Source: CAD feature listing. Evaluate the final solid. Frame: model axes, mm. Face numbers are marked on the shaded views. Coordinates: 2 decimals unless noted, no trailing zeros. Loops run counter-clockwise (first coordinate to the right, second up) from the corner with the lowest first, then second, coordinate; pieces in that order, holes last.
Item 1: Line query: probe 1 along Y at (x, z) = (0, 14.75); probe 2 along Y at (x, z) = (0, 10.75); probe 3 along Y at (x, z) = (-3.5, 9.25). Output: solid intervals per line, ascending.
Item 2: Pull-direction query (Y, two-part tool) for the marked faces 1, 2, 3 and 4; classes: +Y half, -Y half, draft (parallel to the pull), parting line (faces both ways), or undercut.
Item 3: Pin query (flat end, axial travel): pin 1 Ø12.5 at (x, y) = (2, -1.5) entering from +Z; pin 2 Ø2 at (y, z) = (-8.5, 2) entering from +X; pin 3 Ø8 at (y, z) = (-5.5, 10) entering from -X; pin 4 Ø6 at (y, z) = (-6, 9.5) entering from -X. Return the tip coordinate at first contact, or that it passes through.
Item 4: Section query C-C, the plane y = 0. Return the cut outline in (x, z), then the cut area to 3 significant figures.
Item 5: Section query A-A, the plane x = 0. Return the cut outline in (y, z), then the cut area to 3 significant figures.
Item 6: Section query B-B, the plane z = 3.5. Return the cut outline in (x, y), then the cut area to 3 significant figures.
Item 7: Section query D-D, the plane x = -8. Return the cut outline in (y, z), then the cut area to 3 significant figures.
Autodesk Inventor part; units mm, degrees
ref_plane "YZ Plane" through (0, 0, 0) normal (1, 0, 0) x (0, 1, 0)
ref_plane "XZ Plane" through (0, 0, 0) normal (0, 1, 0) x (-1, 0, 0)
ref_plane "XY Plane" through (0, 0, 0) normal (0, 0, 1) x (1, 0, 0)
sketch "Sketch1" plane through (0, 0, 0) normal (0, 0, 1) x (1, 0, 0)
  circle A0 centre (0, 0) radius 5.588
  circle A1 centre (0, 0) radius 4.318
  circle A2 centre (0, 0) radius 14.478
  circle A3 centre (0, 0) radius 15.748
  dimension "d0" = 11.176
  dimension "d1" = 1.27
  dimension "d2" = 8.89
  dimension "d3" = 1.27
extrude "Extrusion1" add sketch "Sketch1" along normal blind 14.478
ref_plane "Work Plane1" through (0, 0, 0) normal (0, 0, -1) x (-1, 0, 0)
sketch "Sketch2" plane through (0, 0, 14.478) normal (0, 0, 1) x (1, 0, 0)
  circle A0 centre (0, 0) radius 15.748
  circle A1 centre (0, 0) radius 14.478
  circle A2 centre (0, 0) radius 5.588
  circle A3 centre (0, 0) radius 4.318
extrude "Extrusion2" add sketch "Sketch2" along normal mid plane 1.27 contours A1
sketch "Sketch3" plane through (0, 0, 15.113) normal (0, 0, 1) x (1, 0, 0)
  circle A0 centre (0, 0) radius 14.478
  arc A1 (-6.0209, 13.1667) -> (6.0209, 13.1667) centre (0, 14.478) ccw
  arc A2 (-14.4131, 1.3691) -> (-8.3923, 11.7976) centre (-12.5383, 7.239) ccw
  arc A3 (-8.3923, -11.7976) -> (-14.4131, -1.3691) centre (-12.5383, -7.239) ccw
  arc A4 (6.0209, -13.1667) -> (-6.0209, -13.1667) centre (0, -14.478) ccw
  arc A5 (14.4131, -1.3691) -> (8.3923, -11.7976) centre (12.5383, -7.239) ccw
  arc A6 (8.3923, 11.7976) -> (14.4131, 1.3691) centre (12.5383, 7.239) ccw
  point P0 (14.4131, 1.3691)
  point P1 (-8.3923, 11.7976)
  point P2 (-14.4131, 1.3691)
  point P3 (-14.4131, -1.3691)
  point P4 (-8.3923, -11.7976)
  point P5 (6.0209, -13.1667)
  point P6 (14.4131, -1.3691)
  dimension "d11" = 360
extrude "Extrusion4" cut sketch "Sketch3" against normal blind 1.27 contours A6 A0 | A0 A5 | A1 A0 | A0 A4 | A2 A0 | A0 A3
properties part number "wheel" material "Iron, Cast"
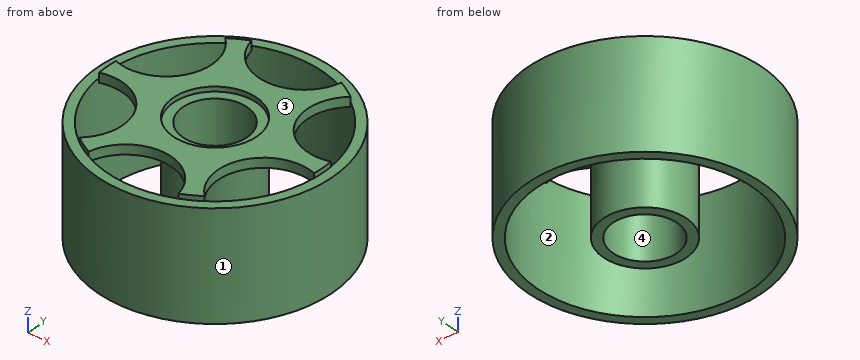
Verdict:
1. probe 1: y = -8.32 to -5.59, 5.59 to 8.32
1. probe 2: y = -15.75 to -14.48, -5.59 to -4.32, 4.32 to 5.59, 14.48 to 15.75
1. probe 3: y = -15.35 to -14.05, -4.36 to -2.53, 2.53 to 4.36, 14.05 to 15.35
2. face 1: parting line
2. face 2: undercut
2. face 3: draft
2. face 4: undercut
3. pin 1: stops at z = 15.11
3. pin 2: stops at x = 13.85
3. pin 3: stops at x = -15.68
3. pin 4: stops at x = -15.46
4. outline: (-15.75, 0) - (-14.48, 0) - (-14.48, 13.84) - (-5.59, 13.84) - (-5.59, 0) - (-4.32, 0) - (-4.32, 14.48) - (-5.59, 14.48) - (-5.59, 15.11) - (-14.48, 15.11) - (-14.48, 14.48) - (-15.75, 14.48) - close; (4.32, 0) - (5.59, 0) - (5.59, 13.84) - (14.48, 13.84) - (14.48, 0) - (15.75, 0) - (15.75, 14.48) - (14.48, 14.48) - (14.48, 15.11) - (5.59, 15.11) - (5.59, 14.48) - (4.32, 14.48) - close
4. area: 96.1 mm2
5. outline: (-15.75, 0) - (-14.48, 0) - (-14.48, 14.48) - (-15.75, 14.48) - close; (-8.32, 13.84) - (-5.59, 13.84) - (-5.59, 0) - (-4.32, 0) - (-4.32, 14.48) - (-5.59, 14.48) - (-5.59, 15.11) - (-8.32, 15.11) - close; (4.32, 0) - (5.59, 0) - (5.59, 13.84) - (8.32, 13.84) - (8.32, 15.11) - (5.59, 15.11) - (5.59, 14.48) - (4.32, 14.48) - close; (14.48, 0) - (15.75, 0) - (15.75, 14.48) - (14.48, 14.48) - close
5. area: 80.5 mm2
6. outline: circle Ø31.5 at (0, 0); circle Ø11.18 at (0, 0); hole circle Ø28.96 at (0, 0); hole circle Ø8.64 at (0, 0)
6. area: 160 mm2
7. outline: (-13.56, 0) - (-12.07, 0) - (-12.07, 13.84) - (-11.41, 13.84) - (-11.41, 15.11) - (-12.07, 15.11) - (-12.07, 14.48) - (-13.56, 14.48) - close; (-3.07, 13.84) - (3.07, 13.84) - (3.07, 15.11) - (-3.07, 15.11) - close; (11.41, 13.84) - (12.07, 13.84) - (12.07, 0) - (13.56, 0) - (13.56, 14.48) - (12.07, 14.48) - (12.07, 15.11) - (11.41, 15.11) - close
7. area: 52.8 mm2
